```python
from build123d import *

# Parameters (mm, degrees)
SKETCH1_R           = 1.6
BOSS_EXTRUDE1_DEPTH = 25


with BuildPart() as part:
    # Sketch1 → Boss-Extrude1 (new body)
    with BuildSketch(Plane(origin=(0, 0, 0), x_dir=(0, 1, 0), z_dir=(0, 0, 1))):
        with BuildLine():
            Line((-18.5, -51.942275653), (-18.5, -54.559600438))
            ThreePointArc((-18.5, -54.559600438), (-18.105910137, -55.75167956), (-17.078947368, -56.473972384))
            ThreePointArc((-17.078947368, -56.473972384), (0, -59), (17.078947368, -56.473972384))
            ThreePointArc((17.078947368, -56.473972384), (18.105910137, -55.75167956), (18.5, -54.559600438))
            Line((18.5, -54.559600438), (18.5, -51.942275653))
            ThreePointArc((18.5, -51.942275653), (17.680887553, -50.328118106), (15.894495413, -50.036137097))
            ThreePointArc((15.894495413, -50.036137097), (0, -52.5), (-15.894495413, -50.036137097))
            ThreePointArc((-15.894495413, -50.036137097), (-17.680887553, -50.328118106), (-18.5, -51.942275653))
        make_face()
        with Locations(Location((-12.5, -54.5, 0), (0, 0, 270))):
            Circle(SKETCH1_R, mode=Mode.SUBTRACT)
        with Locations(Location((12.5, -54.5, 0), (0, 0, 270))):
            Circle(SKETCH1_R, mode=Mode.SUBTRACT)
    extrude(amount=BOSS_EXTRUDE1_DEPTH)


solid = part.part
```
Could you check a few things on this model? Use its own coordinates, in mm. Coordinates: 2 decimals unless noted, no trailing zeros. Write each loop counter-clockwise with the first axis right and the second up, starting at its lowest first coordinate (ties: lowest second). Pieces come first, ordered by that corner, then holes. Notation, with made-up numbers: (89.5, -11) - (111.5, -11) arc R22 ccw to (111.5, 19) - close; hole circle Ø9 at (31, 63.25). An arc over 180 degrees is marked (long way). Use a Markdown table: item, result.
Q1. Imagine slicing it at C-C (x = 53.5). List the corners of the cut face in (y, z) for me.
Geometry check:
| item | result |
|---|---|
| outline | (-18.5, 0) - (-13.75, 0) - (-13.75, 25) - (-18.5, 25) - close; (-11.25, 0) - (11.25, 0) - (11.25, 25) - (-11.25, 25) - close; (13.75, 0) - (18.5, 0) - (18.5, 25) - (13.75, 25) - close |
Q2. Imagine slicing it at D-D (x = 55.5). List the corners of the cut face in (y, z) for me.
Geometry check:
| item | result |
|---|---|
| outline | (-18.27, 0) - (-13.75, 0) - (-13.75, 25) - (-18.27, 25) - close; (-11.25, 0) - (11.25, 0) - (11.25, 25) - (-11.25, 25) - close; (13.75, 0) - (18.27, 0) - (18.27, 25) - (13.75, 25) - close |
Q3. Please list where these lines run through material, in increasing order: L1, parallel to Y at x = 54.5, z = 10; L2, parallel to Y at x = 55.5, z = 5.75; L3, parallel to X at y = 8.5, z = 1.5.
Geometry check:
| item | result |
|---|---|
| L1 | y = -18.5 to -14.1, -10.9 to 10.9, 14.1 to 18.5 |
| L2 | y = -18.27 to -13.75, -11.25 to 11.25, 13.75 to 18.27 |
| L3 | x = 51.81 to 58.38 |
Q4. Imagine slicing it at A-A (y = 11.5). List the corners of the cut face in (x, z) for me (3 decimals), and give its area (3 significant figures).
Geometry check:
| item | result |
|---|---|
| outline | (51.225, 0) - (53.251, 0) - (53.251, 25) - (51.225, 25) - close; (55.749, 0) - (57.868, 0) - (57.868, 25) - (55.749, 25) - close |
| area | 104 mm2 |
Q5. Imagine slicing it at B-B (z = 21). List the corners of the cut face in (x, y) for me, and give its area (3 significant figures).
Geometry check:
| item | result |
|---|---|
| outline | (50.04, -15.89) arc R2 ccw to (51.94, -18.5) - (54.56, -18.5) arc R2 ccw to (56.47, -17.08) arc R59 ccw to (56.47, 17.08) arc R2 ccw to (54.56, 18.5) - (51.94, 18.5) arc R2 ccw to (50.04, 15.89) arc R52.5 cw to start; hole circle Ø3.2 at (54.5, -12.5); hole circle Ø3.2 at (54.5, 12.5) |
| area | 225 mm2 |
Q6. I'm going to push flat-ended pins straight in: pin 1 Ø4 at (y, z) = (3, 10) entering from -X; pin 2 Ø4 at (y, z) = (11.5, 7) entering from -X; pin 3 Ø6 at (y, z) = (-13, 15.5) entering from -X. Where does each tip first touch, or does it pass through?
Geometry check:
| item | result |
|---|---|
| pin 1 | stops at x = 52.26 |
| pin 2 | stops at x = 50.73 |
| pin 3 | stops at x = 50.01 |
Q7. Thinking about a two-plate mould opening in Y: for faces 1 (the cylindrical face through (55.737, -18.117, 12.325)), 2 (the cylindrical face through (56.026, 12.981, 12.325)), 3 (the flat face through (53, 18.5, 12)), which applies, +Y half, -Y half, draft (parallel to the pull), parting line (faces both ways), or undercut?
Geometry check:
| item | result |
|---|---|
| face 1 | -Y half |
| face 2 | undercut |
| face 3 | +Y half |
